Model file for the job. Use its own axes, mm. A direction names the side the tool comes from. Coordinates: 2 decimals unless noted, no trailing zeros. Write each loop counter-clockwise with the first axis right and the second up, starting at its lowest first coordinate (ties: lowest second). Pieces come first, ordered by that corner, then holes. Notation, with made-up numbers: (-28.5, -20.5) -> (-1.5, -20.5) arc R15 cw to (-1.5, -7.5) -> close; hole circle Ø2 at (-17.75, 82.5). An arc over 180 degrees is marked (long way). Write item = value, one per line. Start each with the question number.
from build123d import *

# Parameters (mm, degrees)
SKETCH1_W           = 34
SKETCH1_H           = 30
SKETCH1_R           = 2
BOSS_EXTRUDE1_DEPTH = 30
SKETCH2_W           = 34
SKETCH2_H           = 30
BOSS_EXTRUDE2_DEPTH = 23
SKETCH3_R           = 3.75
CUT_EXTRUDE1_DEPTH  = 30


with BuildPart() as part:
    # Sketch1 → Boss-Extrude1 (new body)
    with BuildSketch(Plane.XY):
        with Locations((17, 15)):
            Rectangle(SKETCH1_W, SKETCH1_H)
        with Locations((4.75, 25.25)):
            Circle(SKETCH1_R, mode=Mode.SUBTRACT)
        with Locations((29.25, 25.25)):
            Circle(SKETCH1_R, mode=Mode.SUBTRACT)
        with Locations((29.25, 4.75)):
            Circle(SKETCH1_R, mode=Mode.SUBTRACT)
        with Locations((4.75, 4.75)):
            Circle(SKETCH1_R, mode=Mode.SUBTRACT)
    extrude(amount=BOSS_EXTRUDE1_DEPTH)

    # Sketch2 → Boss-Extrude2 (add)
    with BuildSketch(Plane.XY.offset(30)):
        with Locations((17, 15)):
            Rectangle(SKETCH2_W, SKETCH2_H)
    extrude(amount=-BOSS_EXTRUDE2_DEPTH)

    # Sketch3 → Cut-Extrude1 (cut)
    with BuildSketch(Plane(origin=(0, 30, 0), x_dir=(1, 0, 0), z_dir=(0, 1, 0))):
        with Locations(Location((17, -15, 0), (0, 0, 270))):
            Circle(SKETCH3_R)
    extrude(amount=-CUT_EXTRUDE1_DEPTH, mode=Mode.SUBTRACT)


solid = part.part
(1) Saw through at A-A (x = 17). Give the cut face in (y, z).
(2) 3-axis set-ups, long thin cutter, end or side, ignore diameter. For faces 5 (the face through (0, 15, 15)), 6 (the face through (5, 5, 7)): which of +Z, -Z, +X, -X, +Y, -Y reach the whole face in a straight line?
(3) Saw through at B-B (y = 4.75). Give the cut face in (x, z).
(4) Saw through at C-C (z = 15). Give the cut face in (x, y), then the cut area to 3 significant figures.
(5) Mould opens along Z. For faces 1 (the face through (17, 15, 30)), 2 (the face through (13, 30, 15)), 3 (the face through (5, 25, 7)), 4 (the face through (13.34, 15.21, 14.19)) say: released by +Z, released by -Z, zero draft, split by the parting line, or undercut.
(6) Drill centre lines: line 1 along X through (y, z) = (4.75, 3.75); line 2 along Y through (x, z) = (4.75, 2.25); line 3 along Y through (x, z) = (30, 4). Where is each one in solid material? Low to high.
(7) Saw through at D-D (x = 4.75). Give the cut face in (y, z), then the cut area to 3 significant figures.
Returned:
q1.outline = (0, 0) -> (30, 0) -> (30, 11.25) -> (0, 11.25) -> close; (0, 18.75) -> (30, 18.75) -> (30, 30) -> (0, 30) -> close
q2.face_5 = +Z, -Z, -X, +Y, -Y
q2.face_6 = -Z
q3.outline = (0, 0) -> (2.75, 0) -> (2.75, 7) -> (6.75, 7) -> (6.75, 0) -> (27.25, 0) -> (27.25, 7) -> (31.25, 7) -> (31.25, 0) -> (34, 0) -> (34, 30) -> (0, 30) -> close; hole circle Ø7.5 at (17, 15)
q4.outline = (0, 0) -> (13.25, 0) -> (13.25, 30) -> (0, 30) -> close; (20.75, 0) -> (34, 0) -> (34, 30) -> (20.75, 30) -> close
q4.area = 795 mm2
q5.face_1 = released by +Z
q5.face_2 = zero draft
q5.face_3 = released by -Z
q5.face_4 = undercut
q6.line_1 = 0 to 2.75, 6.75 to 27.25, 31.25 to 34
q6.line_2 = 0 to 2.75, 6.75 to 23.25, 27.25 to 30
q6.line_3 = 0 to 2.9, 6.6 to 23.4, 27.1 to 30
q7.outline = (0, 0) -> (2.75, 0) -> (2.75, 7) -> (6.75, 7) -> (6.75, 0) -> (23.25, 0) -> (23.25, 7) -> (27.25, 7) -> (27.25, 0) -> (30, 0) -> (30, 30) -> (0, 30) -> close
q7.area = 844 mm2
